```python
from build123d import *

# Parameters (mm, degrees)
F0_W        = 87.5494211584
F0_H        = 66.04
F0_R        = 1.5875
F1_DEPTH    = 3.175
F2_R        = 3.175
F2_R_2      = 1.5875
F3_DEPTH    = 3.175
F4_DEPTH    = 25.4
F5_W        = 87.5494211584
F5_H        = 3.81
F6_DEPTH    = 12.7
F7_T1_DEPTH = 113.6777203162


# Not quite as in the source:
# - a fillet or chamfer that OpenCascade refuses, or shapes differently, is made with other operations: its cross-section is extruded or revolved along the edge and cut away or added


with BuildPart() as f1:
    # F0 (on Top) → F1 (new body)
    with BuildSketch(Plane.XY):
        with Locations((22.1847105792, -24.13)):
            Rectangle(F0_W, F0_H)
        with Locations((-1.27, -48.26)):
            Circle(F0_R, mode=Mode.SUBTRACT)
        with Locations((50.8, -43.18)):
            Circle(F0_R, mode=Mode.SUBTRACT)
        Circle(F0_R, mode=Mode.SUBTRACT)
        with Locations((50.8, -15.24)):
            Circle(F0_R, mode=Mode.SUBTRACT)
    extrude(amount=F1_DEPTH)

    # F2 (on face) → F3 (join)
    with BuildSketch(Plane(origin=(0, 0, 0), x_dir=(1, 0, 0), z_dir=(0, 0, -1))):
        with Locations((9.4847105792, 11.43)):
            Circle(F2_R)
        with Locations((9.4847105792, 11.43)):
            Circle(F2_R_2, mode=Mode.SUBTRACT)
        with Locations((9.4847105792, 36.83)):
            Circle(F2_R)
        with Locations((9.4847105792, 36.83)):
            Circle(F2_R_2, mode=Mode.SUBTRACT)
        with Locations((34.8847105792, 36.83)):
            Circle(F2_R)
        with Locations((34.8847105792, 36.83)):
            Circle(F2_R_2, mode=Mode.SUBTRACT)
        with Locations((34.8847105792, 11.43)):
            Circle(F2_R)
        with Locations((34.8847105792, 11.43)):
            Circle(F2_R_2, mode=Mode.SUBTRACT)
    extrude(amount=F3_DEPTH)

    # F4 (cut): faces of the model
    f4_faces = [f1.faces().sort_by_distance(p)[0] for p in [
        (9.4847105792, -11.43, 0),
        (9.4847105792, -36.83, 0),
        (34.8847105792, -36.83, 0),
        (34.8847105792, -11.43, 0),
    ]]
    extrude(f4_faces, amount=-F4_DEPTH, mode=Mode.SUBTRACT)

    # F5 (on face) → F6 (join)
    with BuildSketch(Plane(origin=(0, 0, 0), x_dir=(1, 0, 0), z_dir=(0, 0, -1))):
        with Locations((22.1847105792, -6.985)):
            Rectangle(F5_W, F5_H)
        with Locations((22.1847105792, 55.245)):
            Rectangle(F5_W, F5_H)
    extrude(amount=F6_DEPTH)

    # F7: chamfer of 5.08 on 4 edges, made by hand

    # F7_s2 → F7_t1 (cut)
    with BuildSketch(Plane.YZ.offset(-34.6541495789)):
        Polygon((8.89, -1.905), (3.81, 3.175), (8.89, 3.175), align=None)
        Polygon((-52.07, 3.175), (-57.15, -1.905), (-57.15, 3.175), align=None)
        Polygon((3.81, -12.7), (8.89, -7.62), (8.89, -12.7), align=None)
        Polygon((-52.07, -12.7), (-57.15, -7.62), (-57.15, -12.7), align=None)
    extrude(amount=F7_T1_DEPTH, mode=Mode.SUBTRACT)


solid = f1.part
```
The listing builds one solid part. Answer for the finished solid, in the listing's coordinates (mm). A direction names the side the tool comes from. Give positions to 0.01 mm unless a question says otherwise; leave off trailing zeros. Write each loop counter-clockwise with the first axis right and the second up, starting at its lowest first coordinate (ties: lowest second). Pieces come first, ordered by that corner, then holes. Notation, with made-up numbers: (25.25, 19) -> (60.25, 19) arc R24 cw to (60.25, 55) -> close; hole circle Ø7 at (51.25, 39). An arc over 180 degrees is marked (long way). Write item = value, one per line. Start each with the question number.
1) The part is cut by section C-C, the plane y = -48.26. Determine the outline of the cut face in (x, z) (1 decimal).
2) The part is cut by section D-D, the plane x = 21.5. Determine the outline of the cut face in (y, z) (3 decimals).
3) Which of the six approach directions +Z, -Z, +X, -X, +Y, -Y give full straight-line access (tool end or side, diameter ignored) to faces 1 (the face through (49.54, -44.146, 1.565)), 2 (the face through (22, -53.34, -6)), 3 (the face through (37.913, -12.384, -1.565))?
4) The part is cut by section A-A, the plane x = 50.8. Count the separate pieces of the cut face and the enclosed holes in it, and give its area (3 significant figures).
5) The part is cut by section B-B, the plane z = -6. Determine the outline of the cut face in (x, y).
6) Each of these flat-tipped pins is pushed along its axis until it touches: pin 1 (5 mm diameter, centred on x = 8.5, y = -10.5, fed in from -Z) (3 decimals); pin 2 (6 mm diameter, centred on x = 34.5, y = -19.5, fed in from -Z). Where does it stop, or does it pass through?
7) Straight lines are drawn through the part: line 1 along X through (y, z) = (-11.43, 1.9); line 2 along X through (y, z) = (-36.83, -0.65); line 3 along Y through (x, z) = (62.5, -5.5). For each, find the intervals that lie inside material, in ascending order.
8) Determine the mould class of faces 4 (the face through (9.071, -14.578, -1.565)), 5 (the face through (21.572, 6.386, 0.599)), 6 (the face through (22, -24, 3.175)) for opening direction Y: +Y half, -Y half, draft (parallel to the pull), parting line (faces both ways), or undercut.
Solutions:
q1.outline = (-21.6, 0) -> (-2.9, 0) -> (-2.9, 3.2) -> (-21.6, 3.2) -> close; (0.3, 0) -> (66, 0) -> (66, 3.2) -> (0.3, 3.2) -> close
q2.outline = (-57.15, -7.62) -> (-53.34, -11.43) -> (-53.34, 0) -> (5.08, 0) -> (5.08, -11.43) -> (8.89, -7.62) -> (8.89, -1.905) -> (3.81, 3.175) -> (-52.07, 3.175) -> (-57.15, -1.905) -> close
q3.face_1 = +Z, -Z
q3.face_2 = -Z, +X, -X
q3.face_3 = -Z
q4.separate_pieces = 3
q4.enclosed_holes = 0
q4.area = 236 mm²
q5.outline = (-21.59, -57.15) -> (65.96, -57.15) -> (65.96, -53.34) -> (-21.59, -53.34) -> close; (-21.59, 5.08) -> (65.96, 5.08) -> (65.96, 8.89) -> (-21.59, 8.89) -> close
q6.pin_1 = -3.175
q6.pin_2 = 0
q7.line_1 = -21.59 to 7.9, 11.07 to 33.3, 36.47 to 65.96
q7.line_2 = 6.31 to 7.9, 11.07 to 12.66, 31.71 to 33.3, 36.47 to 38.06
q7.line_3 = -57.15 to -53.34, 5.08 to 8.89
q8.face_4 = undercut
q8.face_5 = +Y half
q8.face_6 = draft
